Autodesk Fusion 360 part; units mm, degrees
sketch "Sketch1" plane through (0, 0, 0) normal (0, 0, 1) x (1, 0, 0)
  line L0 (-47.9346, 62.0575) -> (-70.9346, 62.0575)
  line L1 (-70.9346, 62.0575) -> (-70.9346, 122.0575)
  line L2 (-70.9346, 122.0575) -> (-47.9346, 122.0575)
  line L3 (-47.9346, 122.0575) -> (-47.9346, 62.0575)
  line L4 (-70.9346, 110) -> (-94.9346, 110)
  line L5 (-94.9346, 110) -> (-94.9346, 75)
  line L6 (-94.9346, 75) -> (-70.9346, 75)
  line L7 (-70.9346, 75) -> (-70.9346, 110)
  dimension "d1" = 35
  dimension "d3" = 60
  dimension "d4" = 24
  dimension "d10" = 23
extrude "Extrude1" add sketch "Sketch1" along normal blind 4
fillet "Fillet1" radius 4 2 edges at (-47.9346, 62.0575, 2) (-47.9346, 122.0575, 2)
fillet "Fillet1" radius 4 2 edges at (-94.9346, 75, 2) (-94.9346, 110, 2)
Verification items for the finished model (mm, model axes). A direction names the side the tool comes from. Coordinates: 2 decimals unless noted, no trailing zeros. Write each loop counter-clockwise with the first axis right and the second up, starting at its lowest first coordinate (ties: lowest second). Pieces come first, ordered by that corner, then holes. Notation, with made-up numbers: M -33.75,66 L -20.75,66 A26 cw -20.75,90 Z; hole C -15.75,-39 d7. An arc over 180 degrees is marked long. Use a Markdown table: item, result.
Q1. Sectioned sample at B-B, the plane y = 117. Record the boundary of the cut face in (x, z).
Reply:
| item | result |
|---|---|
| outline | M -70.93,0 L -47.93,0 L -47.93,4 L -70.93,4 Z |
Q2. Go/stop test with flat-tipped pins: P1, Ø2, axis at x = -77, z = 1, coming from the +Y side; P2, Ø2, axis at y = 116.5, z = 2.5, coming from the -X side; P3, Ø1, axis at y = 76, z = 3, coming from the -X side. Record where each tip stops, or that it passes through.
Reply:
| item | result |
|---|---|
| P1 | stops at y = 110 |
| P2 | stops at x = -70.93 |
| P3 | stops at x = -94.06 |
Q3. Set-up check for faces 1 (the face through (-81, 75, 2)), 2 (the face through (-81, 110, 2)), 3 (the face through (-49.075, 120.855, 2.028)): record each of +Z, -Z, +X, -X, +Y, -Y from which the full face is reachable in a straight line by a thin tool's end or side.
Reply:
| item | result |
|---|---|
| face 1 | +Z, -Z, -X, -Y |
| face 2 | +Z, -Z, -X, +Y |
| face 3 | +Z, -Z, +X, +Y |
Q4. Thickness scan on line 1 (Y direction, x = -71, z = 0.7); line 2 (X direction, y = 111.5, z = 3.8); line 3 (Y direction, x = -51.5, z = 1.05). Record the ranges inside material, lowest first.
Reply:
| item | result |
|---|---|
| line 1 | y = 75 to 110 |
| line 2 | x = -70.93 to -47.93 |
| line 3 | y = 62.08 to 122.03 |
Q5. Sectioned sample at A-A, the plane z = 1.3. Record the boundary of the cut face in (x, y).
Reply:
| item | result |
|---|---|
| outline | M -94.93,79 A4 ccw -90.93,75 L -70.93,75 L -70.93,62.06 L -51.93,62.06 A4 ccw -47.93,66.06 L -47.93,118.06 A4 ccw -51.93,122.06 L -70.93,122.06 L -70.93,110 L -90.93,110 A4 ccw -94.93,106 Z |
Q6. Sectioned sample at C-C, the plane x = -81. Record the boundary of the cut face in (y, z), plus the area to 3 significant figures.
Reply:
| item | result |
|---|---|
| outline | M 75,0 L 110,0 L 110,4 L 75,4 Z |
| area | 140 mm² |
